```python
from build123d import *

# Parameters (mm, degrees)
SKETCH1_W           = 18.5
SKETCH1_H           = 26
BOSS_EXTRUDE1_DEPTH = 1.8
SKETCH2_R           = 2.5
BOSS_EXTRUDE2_DEPTH = 3
SKETCH3_R           = 4
BOSS_EXTRUDE3_DEPTH = 18


with BuildPart() as part:
    # Sketch1 → Boss-Extrude1 (new body)
    with BuildSketch(Plane.XY):
        with Locations((0, 1.5)):
            Rectangle(SKETCH1_W, SKETCH1_H)
    extrude(amount=BOSS_EXTRUDE1_DEPTH)

    # Sketch2 → Boss-Extrude2 (add)
    with BuildSketch(Plane.XY.offset(1.8)):
        with Locations(Location((0, 0, 0), (0, 0, 180))):
            Circle(SKETCH2_R)
    extrude(amount=BOSS_EXTRUDE2_DEPTH)

    # Sketch3 → Boss-Extrude3 (add)
    with BuildSketch(Plane.XY.offset(4.8)):
        Circle(SKETCH3_R)
    extrude(amount=BOSS_EXTRUDE3_DEPTH)


solid = part.part
```
Check sheet for the modelled part. Datum: model origin and axes. Units: mm. A direction names the side the tool comes from. Give positions to 0.01 mm unless a question says otherwise; leave off trailing zeros. Loops run counter-clockwise (first coordinate to the right, second up) from the corner with the lowest first, then second, coordinate; pieces in that order, holes last. Notation, with made-up numbers: (-2.5, -24.75) - (16.5, -24.75) arc R22 ccw to (16.5, -18.75) - close; hole circle Ø8 at (-2, 59). An arc over 180 degrees is marked (long way). One line per question, with ' | ' between items. Start each with the question number.
1. Cross-section at D-D, the plane z = 17.25. Enter the section's corners in (x, y).
2. Cross-section at C-C, the plane y = -3.5. Enter the section's corners in (x, z).
3. Gauge pin test, flat ends, axial feed: pin 1 Ø6 at (x, z) = (1, 7.5) entering from -Y; pin 2 Ø10 at (x, y) = (-4, -1.5) entering from -Z; pin 3 Ø6 at (y, z) = (-6.5, 18.5) entering from -X; pin 4 Ø4 at (y, z) = (4, 20) entering from +X. Record the tip position at first contact, or that the pin passes through.
4. Material ranges on line 1 along Z through (x, y) = (-2.5, 12.5); line 2 along X through (y, z) = (0.25, 14); line 3 along Y through (x, z) = (3, 17.75), recorded low to high. Write a range as [from, to].
5. Draft check along Z on faces 4 (the flat face through (2, 2, 4.8)), 5 (the flat face through (0, 2, 0)), 6 (the flat face through (0, 14.5, 1)). Enter one of: released by +Z, released by -Z, zero draft, split by the parting line, or undercut.
6. Cross-section at A-A, the plane y = 0. Enter the section's corners in (x, z).
7. Cross-section at B-B, the plane x = 0. Enter the section's corners in (y, z), plus the area to 3 significant figures.
8. Set-up check for faces 1 (the cylindrical face through (2.5, -0.1, 3.3)), 2 (the flat face through (0, 0, 22.8)), 3 (the cylindrical face through (-0.867, -3.905, 13.674)): record each of +Z, -Z, +X, -X, +Y, -Y from which the full face is reachable in a straight line by a thin tool's end or side.
Check result:
1) outline: circle Ø8 at (0, 0)
2) outline: (-9.25, 0) - (9.25, 0) - (9.25, 1.8) - (-9.25, 1.8) - close; (-1.94, 4.8) - (1.94, 4.8) - (1.94, 22.8) - (-1.94, 22.8) - close
3) pin 1: stops at y = -4 | pin 2: stops at z = 0 | pin 3: stops at x = -1.94 | pin 4: stops at x = 3.46
4) line 1: z = [0, 1.8] | line 2: x = [-3.99, 3.99] | line 3: y = [-2.65, 2.65]
5) face 4: undercut | face 5: released by -Z | face 6: zero draft
6) outline: (-9.25, 0) - (9.25, 0) - (9.25, 1.8) - (2.5, 1.8) - (2.5, 4.8) - (4, 4.8) - (4, 22.8) - (-4, 22.8) - (-4, 4.8) - (-2.5, 4.8) - (-2.5, 1.8) - (-9.25, 1.8) - close
7) outline: (-11.5, 0) - (14.5, 0) - (14.5, 1.8) - (2.5, 1.8) - (2.5, 4.8) - (4, 4.8) - (4, 22.8) - (-4, 22.8) - (-4, 4.8) - (-2.5, 4.8) - (-2.5, 1.8) - (-11.5, 1.8) - close | area: 206 mm2
8) face 1: none | face 2: +Z, +X, -X, +Y, -Y | face 3: +Z
